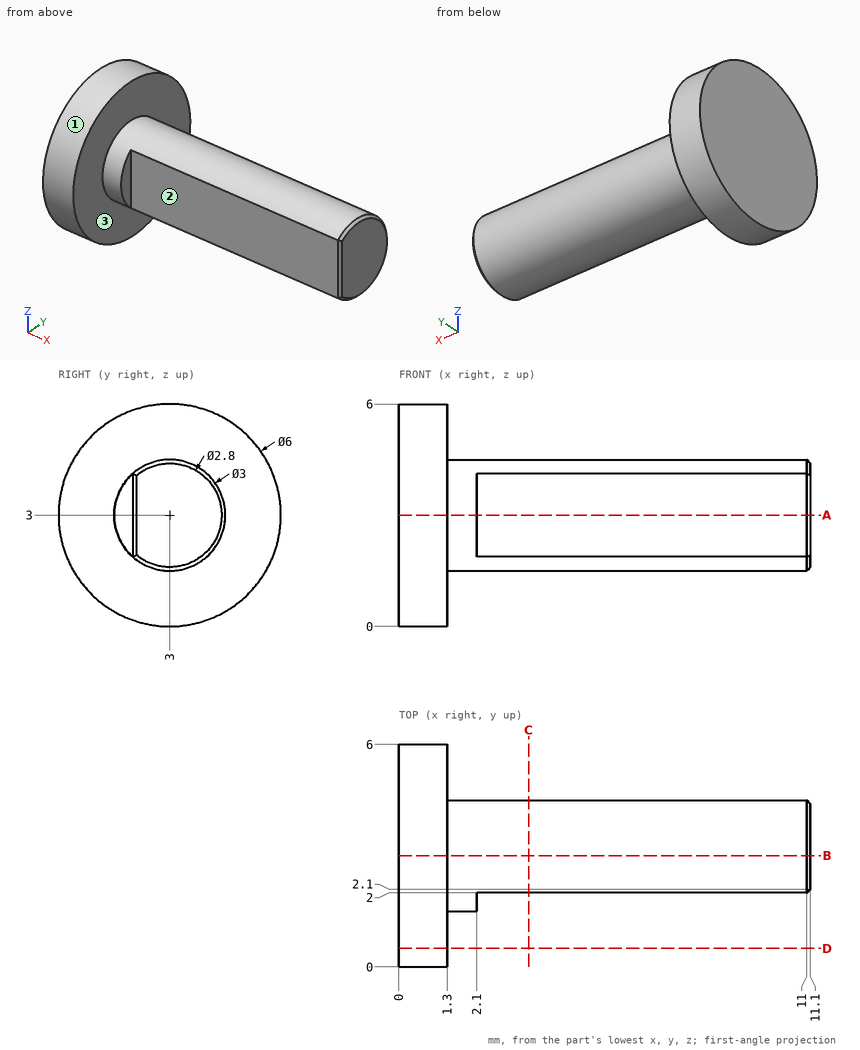
Print and shaded views of the part. All mm, measured from the part's lowest x, y and z. A direction names the side the tool comes from. Coordinates: 2 decimals unless noted, no trailing zeros. Order: outer loops, then holes, each group sorted by start corner. A loop starts at its lowest first (then second) coordinate and runs counter-clockwise, first axis right, second up. Notation, with made-up numbers: M 61,14 L 82,14 A17 cw 82,18 Z; hole C 38,80 d8. An arc over 180 degrees is marked long. Answer as CSV lines item,"result".
1) Cut at A-A (z = 3). List the corners of the cut face in (x, y).
Verdict:
outline,"M 0,0 L 1.3,0 L 1.3,1.5 L 2.1,1.5 L 2.1,2 L 11,2 L 11.1,2.1 L 11.1,4.4 L 11,4.5 L 1.3,4.5 L 1.3,6 L 0,6 Z"
2) Cut at C-C (x = 3.5). List the corners of the cut face in (y, z).
Verdict:
outline,"M 2,1.88 A1.5 ccw long 2,4.12 Z"
3) Drill centre lines: L1, parallel to Z at x = 4.75, y = 3.1; L2, parallel to X at y = 4.75, z = 4.15; L3, parallel to X at y = 1.6, z = 2.7. Where is each one in solid material? Low to high. Write a range as from..to.
Verdict:
L1,"1.5..4.5"
L2,"0..1.3"
L3,"0..2.1"
4) Cut at D-D (y = 0.5). List the corners of the cut face in (x, z).
Verdict:
outline,"M 0,1.34 L 1.3,1.34 L 1.3,4.66 L 0,4.66 Z"
5) Flat gauge pins, fed straight in: P1, Ø3, axis at x = 10, z = 1, coming from the +Y side; P2, Ø0.6, axis at y = 1.5, z = 3.5, coming from the +X side; P3, Ø1.1, axis at x = 8.5, z = 2.5, coming from the -Y side. Where does each tip first touch, or does it go through?
Verdict:
P1,"y = 4.41"
P2,"x = 2.1"
P3,"y = 2"
6) Cut at B-B (y = 3). List the corners of the cut face in (x, z).
Verdict:
outline,"M 0,0 L 1.3,0 L 1.3,1.5 L 11,1.5 L 11.1,1.6 L 11.1,4.4 L 11,4.5 L 1.3,4.5 L 1.3,6 L 0,6 Z"
7) 3-axis set-ups, long thin cutter, end or side, ignore diameter. For the marked faces 1, 2 and 3: which of +Z, -Z, +X, -X, +Y, -Y reach the whole face in a straight line?
Verdict:
face 1,"+X, -X"
face 2,"+Z, -Z, +X, -Y"
face 3,"+X"
